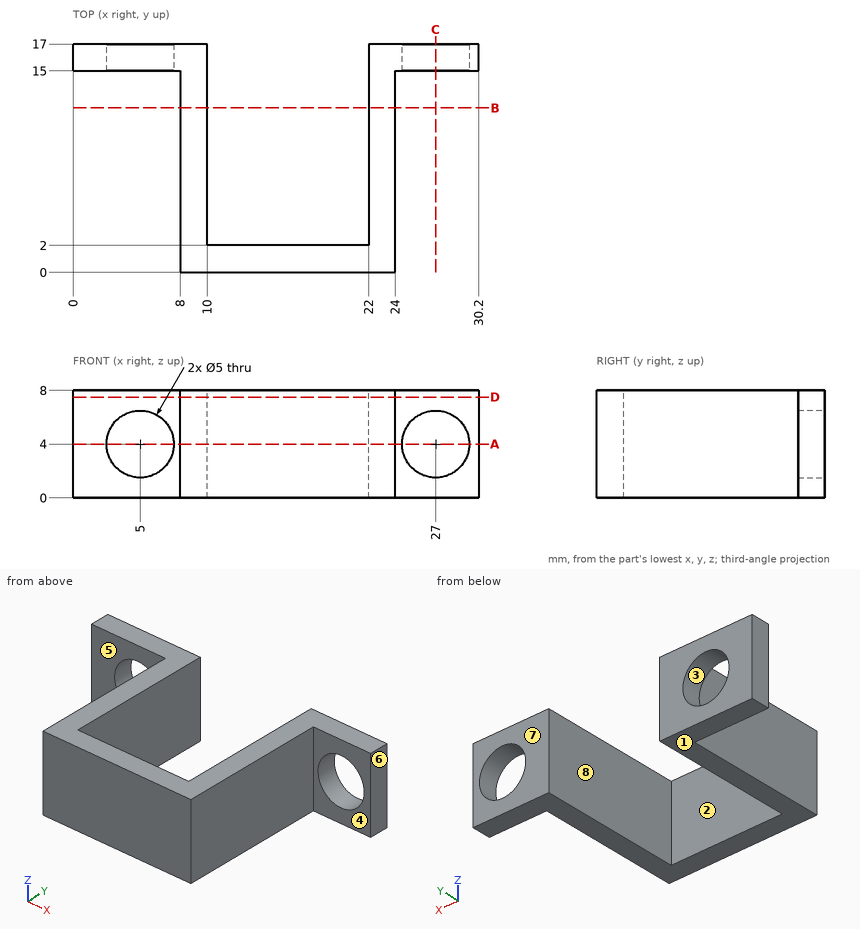
Geometry: see drawing. Coordinates: mm, zero at the bounding-box minimum. A direction names the side the tool comes from. Coordinates: 2 decimals unless noted, no trailing zeros. Loops run counter-clockwise (first coordinate to the right, second up) from the corner with the lowest first, then second, coordinate; pieces in that order, holes last. Notation, with made-up numbers: (14.25, -39.5) - (27.25, -39.5) arc R23 cw to (27.25, -24.5) - close; hole circle Ø7 at (80, 52). An arc over 180 degrees is marked (long way). Answer in a Markdown table with one row per item.
(1) Mould query, pull axis Z, two halves, no side actions, for the marked faces 1, 2 and 3. Classes: pulls with the +Z half, pulls with the -Z half, needs draft (parallel to the pull), parting line crosses it, or undercut.
Model answer:
| item | result |
|---|---|
| face 1 | pulls with the -Z half |
| face 2 | needs draft |
| face 3 | undercut |
(2) Cut plane D-D on z = 7.5. Output: boundary loops of the cut face in (x, y).
Model answer:
| item | result |
|---|---|
| outline | (0, 15) - (8, 15) - (8, 0) - (24, 0) - (24, 15) - (30.2, 15) - (30.2, 17) - (22, 17) - (22, 2) - (10, 2) - (10, 17) - (0, 17) - close |
(3) Pin query (flat end, axial travel): P1, Ø4.5, axis at x = 5, z = 4, coming from the -Y side; P2, Ø10, axis at x = 26.5, y = 12, coming from the -Z side; P3, Ø2.5, axis at y = 6.5, z = 3, coming from the +X side; P4, Ø3, axis at x = 26.5, z = 3, coming from the -Y side. Return the tip coordinate at first contact, or that it passes through.
Model answer:
| item | result |
|---|---|
| P1 | passes through |
| P2 | stops at z = 0 |
| P3 | stops at x = 24 |
| P4 | stops at y = 15 |
(4) Cut plane A-A on z = 4. Output: boundary loops of the cut face in (x, y).
Model answer:
| item | result |
|---|---|
| outline | (0, 15) - (2.5, 15) - (2.5, 17) - (0, 17) - close; (7.5, 15) - (8, 15) - (8, 0) - (24, 0) - (24, 15) - (24.5, 15) - (24.5, 17) - (22, 17) - (22, 2) - (10, 2) - (10, 17) - (7.5, 17) - close; (29.5, 15) - (30.2, 15) - (30.2, 17) - (29.5, 17) - close |
(5) Set-up query: the marked faces 4, 5, 6, 7 and 8. Return all of +Z, -Z, +X, -X, +Y, -Y with unobstructed straight access to the full face (end or side cutting, diameter ignored); none if empty.
Model answer:
| item | result |
|---|---|
| face 4 | +Z, -Z, +X, -Y |
| face 5 | +Z, -Z, -X, -Y |
| face 6 | +Z, -Z, +X, +Y, -Y |
| face 7 | +Z, -Z, +X, -X, +Y |
| face 8 | +Z, -Z, +Y |
(6) Cut plane B-B on y = 12.25. Output: boundary loops of the cut face in (x, z), plus the area to 3 significant figures.
Model answer:
| item | result |
|---|---|
| outline | (8, 0) - (10, 0) - (10, 8) - (8, 8) - close; (22, 0) - (24, 0) - (24, 8) - (22, 8) - close |
| area | 32.0 mm² |
(7) Material intervals for L1, parallel to X at y = 16.3, z = 4; L2, parallel to Z at x = 5, y = 16.1; L3, parallel to X at y = 6, z = 1, sorted ascending. Write a range as from..to.
Model answer:
| item | result |
|---|---|
| L1 | x = 0..2.5, 7.5..10, 22..24.5, 29.5..30.2 |
| L2 | z = 0..1.5, 6.5..8 |
| L3 | x = 8..10, 22..24 |
(8) Cut plane C-C on x = 27. Output: boundary loops of the cut face in (y, z).
Model answer:
| item | result |
|---|---|
| outline | (15, 0) - (17, 0) - (17, 1.5) - (15, 1.5) - close; (15, 6.5) - (17, 6.5) - (17, 8) - (15, 8) - close |
